The model under review builds one solid part; all positions refer to its coordinate system, in mm. Face numbers are marked on the shaded views. Coordinates: 2 decimals unless noted, no trailing zeros. Order: outer loops, then holes, each group sorted by start corner. A loop starts at its lowest first (then second) coordinate and runs counter-clockwise, first axis right, second up. Notation, with made-up numbers: M 78.5,-15 L 133.5,-15 A15 cw 133.5,2 Z; hole C 67.25,0.5 d8. An arc over 180 degrees is marked long. One line per item, written item: value.
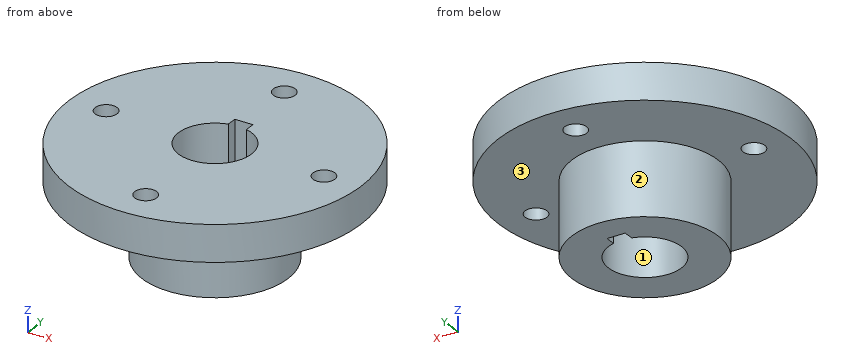
```python
from build123d import *

# Parameters (mm, degrees)
SKETCH1_R           = 200
BOSS_EXTRUDE1_DEPTH = 50
SKETCH2_R           = 100
BOSS_EXTRUDE2_DEPTH = 100
SKETCH3_R           = 15
CUT_EXTRUDE1_DEPTH  = 321.156211872
SKETCH4_R           = 50
CUT_EXTRUDE2_DEPTH  = 321.156211872
SKETCH5_W           = 25
SKETCH5_H           = 25
CUT_EXTRUDE3_DEPTH  = 321.156211872


with BuildPart() as part:
    # Sketch1 → Boss-Extrude1 (new body)
    with BuildSketch(Plane.XY):
        Circle(SKETCH1_R)
    extrude(amount=BOSS_EXTRUDE1_DEPTH)

    # Sketch2 → Boss-Extrude2 (add)
    with BuildSketch(Plane(origin=(0, 0, 0), x_dir=(-1, 0, 0), z_dir=(0, 0, -1))):
        with Locations(Location((0, 0, 0), (0, 0, 180))):
            Circle(SKETCH2_R)
    extrude(amount=BOSS_EXTRUDE2_DEPTH)

    # Sketch3 → Cut-Extrude1 (cut, through all)
    with BuildSketch(Plane.XY.offset(50)):
        with Locations((0, 150)):
            Circle(SKETCH3_R)
        with Locations((150, 0)):
            Circle(SKETCH3_R)
        with Locations((0, -150)):
            Circle(SKETCH3_R)
        with Locations((-150, 0)):
            Circle(SKETCH3_R)
    extrude(amount=-CUT_EXTRUDE1_DEPTH, mode=Mode.SUBTRACT)

    # Sketch4 → Cut-Extrude2 (cut, through all)
    with BuildSketch(Plane.XY.offset(50)):
        Circle(SKETCH4_R)
    extrude(amount=-CUT_EXTRUDE2_DEPTH, mode=Mode.SUBTRACT)

    # Sketch5 → Cut-Extrude3 (cut, through all)
    with BuildSketch(Plane.XY.offset(50)):
        with Locations((0, 50)):
            Rectangle(SKETCH5_W, SKETCH5_H)
    extrude(amount=-CUT_EXTRUDE3_DEPTH, mode=Mode.SUBTRACT)


solid = part.part
```
(1) For L1, parallel to Y at x = 0, z = 10; L2, parallel to Z at x = 93, y = -135.5; L3, parallel to Y at x = -150, z = 24, list the stretches that pass through material, from the lowest coordinate up.
Geometry results:
L1: y = -200 to -165, -135 to -50, 62.5 to 135, 165 to 200
L2: z = 0 to 50
L3: y = -132.29 to -15, 15 to 132.29
(2) We need section D-D, the plane z = -16. State the section outline as (x, y) points, plus the area to 3 significant figures.
Geometry results:
outline: C 0,0 d200; hole M -12.5,48.41 A50 ccw long 12.5,48.41 L 12.5,62.5 L -12.5,62.5 Z
area: 23,200 mm2
(3) We need section B-B, the plane x = 0. State the section outline as (y, z) points.
Geometry results:
outline: M -200,0 L -165,0 L -165,50 L -200,50 Z; M -135,0 L -100,0 L -100,-100 L -50,-100 L -50,50 L -135,50 Z; M 62.5,-100 L 100,-100 L 100,0 L 135,0 L 135,50 L 62.5,50 Z; M 165,0 L 200,0 L 200,50 L 165,50 Z
(4) Insertion check: pin 1 Ø5 at (x, y) = (-151.5, -12) entering from +Z; pin 2 Ø12 at (y, z) = (18, -44) entering from -X; pin 3 Ø8 at (x, y) = (-37, 132) entering from -Z; pin 4 Ø4 at (y, z) = (58, -23.5) entering from -X. Each pin has a flat end and moves straight along its axis. Give the tip position at first contact, or say it passes through.
Geometry results:
pin 1: passes through
pin 2: stops at x = -99.28
pin 3: stops at z = 0
pin 4: stops at x = -82.85
(5) We need section A-A, the plane y = 0. State the section outline as (x, z) points.
Geometry results:
outline: M -200,0 L -165,0 L -165,50 L -200,50 Z; M -135,0 L -100,0 L -100,-100 L -50,-100 L -50,50 L -135,50 Z; M 50,-100 L 100,-100 L 100,0 L 135,0 L 135,50 L 50,50 Z; M 165,0 L 200,0 L 200,50 L 165,50 Z
(6) We need section C-C, the plane y = -150. State the section outline as (x, z) points, plus the area to 3 significant figures.
Geometry results:
outline: M -132.29,0 L -15,0 L -15,50 L -132.29,50 Z; M 15,0 L 132.29,0 L 132.29,50 L 15,50 Z
area: 11,700 mm2
(7) Mouldability with a two-part tool opening along Y and no side actions: class the marked faces 1, 2 and 3 as +Y half, -Y half, draft (parallel to the pull), parting line (faces both ways), or undercut.
Geometry results:
face 1: undercut
face 2: parting line
face 3: draft
